```python
from build123d import *

# Parameters (mm, degrees)
SKETCH_1_R          = 9.5
SKETCH_1_R_2        = 4
EXTRUDE_1_DEPTH     = 3
SKETCH_2_R          = 8.25
SKETCH_2_R_2        = 5.15
CUT_EXTRUDE_2_DEPTH = 0.2
FILLET_1_R          = 0.3


with BuildPart() as part:
    # 草图1 → 拉伸1 (new, symmetric)
    with BuildSketch(Plane.XY):
        Circle(SKETCH_1_R)
        Circle(SKETCH_1_R_2, mode=Mode.SUBTRACT)
    extrude(amount=EXTRUDE_1_DEPTH, both=True)

    # 草图2 → 拉伸2 (cut)
    with BuildSketch(Plane.XY.offset(3)):
        Circle(SKETCH_2_R)
        Circle(SKETCH_2_R_2, mode=Mode.SUBTRACT)
    cut_extrude_2 = extrude(amount=-CUT_EXTRUDE_2_DEPTH, mode=Mode.SUBTRACT)

    # 镜向1: 拉伸2 across plane
    add(cut_extrude_2.mirror(Plane.XY), mode=Mode.SUBTRACT)

    # 圆角1
    fillet_1_edges = [part.edges().sort_by_distance(p)[0] for p in [
        (-9.5, 0, -3),
        (-9.5, 0, 3),
        (-4, 0, -3),
        (-4, 0, 3),
    ]]
    fillet(fillet_1_edges, radius=FILLET_1_R)


solid = part.part
```
Verification items for the finished model (mm, model axes). A direction names the side the tool comes from. Give positions to 0.01 mm unless a question says otherwise; leave off trailing zeros. Order: outer loops, then holes, each group sorted by start corner. A loop starts at its lowest first (then second) coordinate and runs counter-clockwise, first axis right, second up. Notation, with made-up numbers: M 2.5,30.5 L 28.5,30.5 A23 cw 28.5,55.5 Z; hole C -12.75,4.25 d2. An arc over 180 degrees is marked long. Return JSON: item names as keys, results as strings. Group by question number.
1) Mould release check, pull along Y, two halves, no side actions. Record for faces 1 (the face through (-4, -4, 2.8)), 2 (the face through (2, -4, -3)), 3 (the face through (4.38, -8.43, 0.04)), 4 (the face through (-0.867, -3.905, -0.038)): pulls with the +Y half, pulls with the -Y half, needs draft (parallel to the pull), parting line crosses it, or undercut.
2) Access from +Z, -Z, +X, -X, +Y, -Y to the whole of each face (thin tool, end or side, straight path). Record for faces 5 (the face through (-4, -4, -2.8)), 6 (the face through (-3, 8, 3)).
3) Scan lines: line 1 (Y direction, x = 0, z = -0.9); line 2 (Y direction, x = 0, z = -2.9); line 3 (Z direction, x = 1.25, y = 6.5). Record each from-to range of solid material in increasing order.
4) Section check C-C on z = 0.3. Record the cut outline in (x, y), and give its area (3 significant figures).
5) Go/stop test with flat-tipped pins: pin 1 Ø2 at (x, z) = (-2, -1) entering from -Y; pin 2 Ø3 at (x, z) = (-6, 2) entering from +Y; pin 3 Ø3 at (x, z) = (7, -1.5) entering from -Y. Record where each tip stops, or that it passes through.
Answer block:
{
 "1": {"face 1": "undercut", "face 2": "needs draft", "face 3": "parting line crosses it", "face 4": "undercut"},
 "2": {"face 5": "-Z", "face 6": "+Z, +X, -X, +Y, -Y"},
 "3": {"line 1": "y = -9.5 to -4, 4 to 9.5", "line 2": "y = -9.42 to -8.25, -5.15 to -4.08, 4.08 to 5.15, 8.25 to 9.42", "line 3": "z = -2.8 to 2.8"},
 "4": {"outline": "C 0,0 d19; hole C 0,0 d8", "area": "233 mm^2"},
 "5": {"pin 1": "stops at y = -9.45", "pin 2": "stops at y = 8.37", "pin 3": "stops at y = -7.75"}
}
